Autodesk Inventor part; units mm, degrees
ref_plane "YZ Plane" through (0, 0, 0) normal (1, 0, 0) x (0, 1, 0)
ref_plane "XZ Plane" through (0, 0, 0) normal (0, 1, 0) x (-1, 0, 0)
ref_plane "XY Plane" through (0, 0, 0) normal (0, 0, 1) x (1, 0, 0)
sketch "Sketch1" plane through (0, 0, 0) normal (1, 0, 0) x (0, 1, 0)
  line L0 (0, 0) -> (15, 0)
  line L1 (15, 0) -> (15, -15)
  line L2 (15, -15) -> (0, -15)
  line L3 (0, -15) -> (0, 0)
  dimension "d1" = 15
  dimension "d2" = 15
extrude "Extrusion1" add sketch "Sketch1" along normal blind 165
sketch "Sketch2" plane through (0, 0, 0) normal (0, 0, 1) x (1, 0, 0)
  line L0 (104.748, 28) -> (222.799, 28) construction
  line L1 (0, 15) -> (165, 15)
  line L2 (165, 15) -> (165, 0)
  line L3 (165, 15) -> (165, 53.4623) construction
  line L4 (116.7358, 25) -> (195.5126, 25) construction
  line L5 (0, 0) -> (165, 0)
  line L6 (176.2583, 34.5) -> (185.2344, 39.6823)
  arc A0 (165, 0) -> (185.2344, 39.6823) centre (165, 25) ccw
  arc A1 (165, 15) -> (176.2583, 34.5) centre (165, 28) ccw
  dimension "d5" = 13
  dimension "d6" = 25
  dimension "d9" = 11.2583
  dimension "d10" = 20.2344
extrude "Extrusion2" add sketch "Sketch2" against normal blind 15
sketch "Sketch3" plane through (0, 0, 0) normal (0, 0, 1) x (1, 0, 0)
  line L0 (0, 0) -> (165, 0)
  point P0 (45, 7.5)
hole "Hole1" at (45, 7.5, 0) direction (0, 0, -1) diameter 6 end through all
properties part number "garra"
Here's how the part is built. I have some questions about the finished solid (model axes, mm). A direction names the side the tool comes from. Give positions to 0.01 mm unless a question says otherwise; leave off trailing zeros. Loops run counter-clockwise (first coordinate to the right, second up) from the corner with the lowest first, then second, coordinate; pieces in that order, holes last. Notation, with made-up numbers: (39, 2.25) -> (71, 2.25) arc R5 cw to (71, 10.25) -> close; hole circle Ø8 at (-26.5, -13.5). An arc over 180 degrees is marked (long way). Answer as a JSON object with one key per item and string values. Group by question number.
Item 1: Thinking about a two-plate mould opening in Y: for faces 3 (the flat face through (180.684, 37.055, -7.395)), 4 (the cylindrical face through (176.162, 21.336, -7.395)), 5 (the flat face through (115, 11, -15)), which applies, pulls with the +Y half, pulls with the -Y half, needs draft (parallel to the pull), parting line crosses it, or undercut?
Item 2: On a 3-axis mill with a long thin cutter (end or side, diameter ignored), from which of +Z, -Z, +X, -X, +Y, -Y can I reach the whole of each face in a straight line? I mean faces 1 (the flat face through (81, 15, -7)), 2 (the flat face through (115, 11, 0)). Say none if no direction works.
Item 3: Will these pins go through, and if not, where does the flat tip stop? pin 1 (5 mm diameter, centred on x = 45, y = 7.5, fed in from -Z); pin 2 (6 mm diameter, centred on y = 5, z = -9, fed in from +X); pin 3 (7.5 mm diameter, centred on x = 74, z = -7.5, fed in from +Y); pin 4 (1 mm diameter, centred on y = 28, z = -10.5, fed in from -X).
Item 4: Imagine slicing it at A-A on z = -11. Write out the boundary of the cut face in (x, y).
Item 5: I need wall thicknesses on L1, parallel to Y at x = 45, z = -6; L2, parallel to Y at x = 21.5, z = -2.5; L3, parallel to X at y = 7.5, z = -7.25. Which ranges of each line are inside material? Lowest first, please.
Item 6: Imagine slicing it at C-C on y = 7.5. Write out the boundary of the cut face in (x, z).
Item 7: Imagine slicing it at D-D on x = 139. Write out the boundary of the cut face in (y, z).
Item 8: Imagine slicing it at B-B on x = 45. Write out the boundary of the cut face in (y, z), then the cut area to 3 significant figures.
Answer list:
{
 "1": {"face 3": "pulls with the +Y half", "face 4": "undercut", "face 5": "needs draft"},
 "2": {"face 1": "+Z, -Z, -X, +Y", "face 2": "+Z, +X, -X, +Y, -Y"},
 "3": {"pin 1": "passes through", "pin 2": "stops at x = 183.33", "pin 3": "stops at y = 15", "pin 4": "stops at x = 177.99"},
 "4": {"outline": "(0, 0) -> (165, 0) arc R25 ccw to (185.23, 39.68) -> (176.26, 34.5) arc R13 cw to (165, 15) -> (0, 15) -> close; hole circle Ø6 at (45, 7.5)"},
 "5": {"L1": "y = 0 to 4.5, 10.5 to 15", "L2": "y = 0 to 15", "L3": "x = 0 to 42, 48 to 182.85"},
 "6": {"outline": "(0, -15) -> (42, -15) -> (42, 0) -> (0, 0) -> close; (48, -15) -> (182.85, -15) -> (182.85, 0) -> (48, 0) -> close"},
 "7": {"outline": "(0, -15) -> (15, -15) -> (15, 0) -> (0, 0) -> close"},
 "8": {"outline": "(0, -15) -> (4.5, -15) -> (4.5, 0) -> (0, 0) -> close; (10.5, -15) -> (15, -15) -> (15, 0) -> (10.5, 0) -> close", "area": "135 mm2"}
}
